Autodesk Inventor part; units mm, degrees
ref_plane "YZ Plane" through (0, 0, 0) normal (1, 0, 0) x (0, 1, 0)
ref_plane "XZ Plane" through (0, 0, 0) normal (0, 1, 0) x (-1, 0, 0)
ref_plane "XY Plane" through (0, 0, 0) normal (0, 0, 1) x (1, 0, 0)
sketch "Sketch1" plane through (0, 0, 0) normal (0, 0, 1) x (1, 0, 0)
  line L0 (-25, 0) -> (25, 0)
  line L1 (25, 0) -> (25, 394)
  line L2 (25, 394) -> (-25, 394)
  line L3 (-25, 394) -> (-25, 0)
  point P0 (0, 0)
  point P1 (0, 0)
  dimension "d0" = 394
  dimension "d1" = 50
extrude "Extrusion1" add sketch "Sketch1" along normal blind 3
sketch "Sketch2" plane through (0, 0, 0) normal (0, 0, -1) x (-1, 0, 0)
  line L0 (-22, 334) -> (-25, 334)
  line L1 (-22, 374) -> (-25, 374)
  line L2 (-22, 374) -> (-22, 354)
  line L3 (-25, 334) -> (-25, 354)
  line L4 (-25, 0) -> (-25, 394)
  line L5 (-22, 354) -> (-25, 354)
  line L6 (-25, 0) -> (-25, 394)
  line L7 (-25, 394) -> (25, 394)
  line L8 (-25, 354) -> (-25, 374)
  line L9 (-22, 354) -> (-22, 334)
  line L10 (-22, 374) -> (-25, 374)
  line L11 (-25, 374) -> (-25, 394)
  line L12 (-25, 394) -> (-22, 394)
  line L13 (-22, 394) -> (-22, 374)
  point P0 (0, 0)
  dimension "d4" = 20
  dimension "d10" = 20
  dimension "d55" = 60
  dimension "d56" = 20
extrude "Extrusion2" cut sketch "Sketch2" against normal blind 3 contours L5 L4 L1 L2 | L1 L4 L7 L13
sketch "Sketch3" plane through (0, 0, 0) normal (0, 0, -1) x (-1, 0, 0)
  line L0 (-25, 0) -> (-25, 354)
  line L1 (-25, 354) -> (-31, 354)
  line L2 (-31, 354) -> (-31, 336)
  line L3 (-29, 334) -> (-25, 334)
  line L4 (-25, 334) -> (-25, 354)
  line L5 (-31, 354) -> (-25, 354)
  line L6 (-25, 354) -> (-25, 374)
  line L7 (-25, 374) -> (-28, 374)
  line L8 (-31, 364) -> (-31, 354)
  line L9 (-31, 364) -> (-28, 374)
  line L10 (-28, 374) -> (-31, 374) construction
  arc A0 (-31, 336) -> (-29, 334) centre (-29, 336) ccw
  point P0 (0, 0)
  point P1 (-31, 334)
  dimension "d11" = 20
  dimension "d12" = 20
  dimension "d13" = 6
  dimension "d16" = 2
extrude "Extrusion3" add sketch "Sketch3" against normal blind 3
pattern_linear "Rectangular Pattern1" count 3 spacing 120 along (0, -1, 0) of "Extrusion2", "Extrusion3"
mirror "Mirror1" about plane through (0, 0, 0) normal (1, 0, 0) of "Extrusion2", "Rectangular Pattern1", "Extrusion3"
sketch "Sketch4" plane through (0, 0, 0) normal (0, 0, -1) x (-1, 0, 0)
  line L0 (-22, 384) -> (18.49, 384) construction
  line L1 (-22, 394) -> (22, 394)
  line L2 (-22, 394) -> (-22, 354)
  point P0 (0, 0)
  point P1 (-8, 384)
  point P2 (8, 384)
  dimension "d17" = 16
  dimension "d52" = 10
  dimension "d53" = 14
hole "Hole1" at (8, 384, 0) at (-8, 384, 0) direction (0, 0, 1) diameter 3.2 end through all
sketch "Sketch5" plane through (0, 0, 0) normal (0, 0, -1) x (-1, 0, 0)
  line L0 (-10, 0) -> (10, 0)
  line L1 (-10, 0) -> (-10, -6)
  line L2 (10, -6) -> (-10, -6)
  line L3 (10, 0) -> (10, -6)
  line L4 (25, 94) -> (25, 0)
  point P0 (0, 0)
  dimension "d48" = 6
  dimension "d50" = 20
  dimension "d51" = 15
extrude "Extrusion4" add sketch "Sketch5" against normal blind 3
sketch "Sketch6" plane through (0, 0, 0) normal (0, 0, -1) x (-1, 0, 0)
  line L0 (0, 36.6667) -> (0, 53.3333) construction
  line L1 (-10, 36.6667) -> (-10, 53.3333)
  line L2 (10, 53.3333) -> (10, 36.6667)
  arc A0 (-10, 36.6667) -> (10, 36.6667) centre (0, 36.6667) ccw
  arc A1 (10, 53.3333) -> (-10, 53.3333) centre (0, 53.3333) ccw
  line L3 (0, 343.6331) -> (0, 309.773) construction
  line L4 (-5.8349, 343.6331) -> (-5.8349, 309.773)
  line L5 (5.8349, 309.773) -> (5.8349, 343.6331)
  arc A2 (5.8349, 343.6331) -> (-5.8349, 343.6331) centre (0, 343.6331) ccw
  arc A3 (-5.8349, 309.773) -> (5.8349, 309.773) centre (0, 309.773) ccw
  line L6 (0, 243.6331) -> (0, 209.773) construction
  line L7 (-5.8349, 243.6331) -> (-5.8349, 209.773)
  line L8 (5.8349, 209.773) -> (5.8349, 243.6331)
  arc A4 (5.8349, 243.6331) -> (-5.8349, 243.6331) centre (0, 243.6331) ccw
  arc A5 (-5.8349, 209.773) -> (5.8349, 209.773) centre (0, 209.773) ccw
  line L9 (0, 143.6331) -> (0, 109.773) construction
  line L10 (-5.8349, 143.6331) -> (-5.8349, 109.773)
  line L11 (5.8349, 109.773) -> (5.8349, 143.6331)
  arc A6 (5.8349, 143.6331) -> (-5.8349, 143.6331) centre (0, 143.6331) ccw
  arc A7 (-5.8349, 109.773) -> (5.8349, 109.773) centre (0, 109.773) ccw
  point P0 (0, 0)
  point P1 (0, 45)
  point P2 (0, 326.7031)
  point P3 (0, 226.7031)
  point P4 (0, 126.7031)
  dimension "d28" = 10
  dimension "d29" = 45
  dimension "d43" = 100
extrude "Extrusion5" cut sketch "Sketch6" against normal blind 3
sketch "Sketch7" plane through (0, 0, 0) normal (0, 0, -1) x (-1, 0, 0)
  line L0 (-22, 10) -> (26.4852, 10) construction
  line L1 (-25, 0) -> (-25, 94)
  line L2 (-10, 0) -> (-25, 0)
  point P0 (0, 0)
  point P1 (-8, 10)
  point P2 (8, 10)
  dimension "d32" = 16
  dimension "d33" = 17
  dimension "d54" = 10
hole "Hole2" at (8, 10, 0) at (-8, 10, 0) direction (0, 0, 1) diameter 3.2 end through all
properties part number "Camera mounting back"
Geometry: final body of the model. Coordinates: model frame, mm. A direction names the side the tool comes from. Give positions to 0.01 mm unless a question says otherwise; leave off trailing zeros. Order: outer loops, then holes, each group sorted by start corner. A loop starts at its lowest first (then second) coordinate and runs counter-clockwise, first axis right, second up. Notation, with made-up numbers: (80.25, -4) -> (85.25, -4) arc R16 ccw to (85.25, 3) -> close; hole circle Ø1 at (85, -17). An arc over 180 degrees is marked (long way). Write each question's results on one line, items separated by ' | '. Start each with the question number.
1) First-contact query: pin 1 (1.5 mm diameter, centred on x = 24, z = 1.5, fed in from +Y); pin 2 (0.9 mm diameter, centred on x = 26, z = 1.5, fed in from +Y); pin 3 (2.5 mm diameter, centred on x = -8, y = 384, fed in from +Z). Flat tips, straight axial feed; report the tip coordinate or a pass-through.
2) Section C-C (y = 369.5). Return loops of the section in (x, z).
3) Section B-B (y = 327). Return loops of the section in (x, z).
4) Set-up query: faces 3 (the cylindrical face through (0.22, 26.67, 1.48)), 4 (the flat face through (0, 197, 3)). Return all of +Z, -Z, +X, -X, +Y, -Y with unobstructed straight access to the full face (end or side cutting, diameter ignored); none if empty.
5) Line query: line 1 (Y direction, x = 24, z = 2); line 2 (X direction, y = 10, z = 1.6); line 3 (X direction, y = 384, z = 1.7). Output: solid intervals per line, ascending. Write a range as from..to.
6) Section D-D (z = 1.2). Count the separate pieces of the cut face and the enclosed holes in it, then the cut area to 3 significant figures.
7) Section A-A (x = 0). Return loops of the section in (y, z).
8) Draft query along Y for faces 1 (the flat face through (0, 197, 0)), 2 (the cylindrical face through (-0.22, 63.33, 1.48)). Return one class per face: pulls with the +Y half, pulls with the -Y half, needs draft (parallel to the pull), parting line crosses it, or undercut.
Calculated:
1) pin 1: y = 354 | pin 2: y = 374 | pin 3: through
2) outline: (-29.35, 0) -> (-25, 0) -> (-25, 3) -> (-29.35, 3) -> close; (-22, 0) -> (22, 0) -> (22, 3) -> (-22, 3) -> close; (25, 0) -> (29.35, 0) -> (29.35, 3) -> (25, 3) -> close
3) outline: (-25, 0) -> (-5.83, 0) -> (-5.83, 3) -> (-25, 3) -> close; (5.83, 0) -> (25, 0) -> (25, 3) -> (5.83, 3) -> close
4) face 3: +Z, -Z | face 4: +Z, +X, -X, +Y, -Y
5) line 1: 0..114, 154..234, 274..354 | line 2: -25..-9.6, -6.4..6.4, 9.6..25 | line 3: -22..-9.6, -6.4..6.4, 9.6..22
6) separate pieces: 1 | enclosed holes: 8 | area: 18,300 mm2
7) outline: (-6, 0) -> (26.67, 0) -> (26.67, 3) -> (-6, 3) -> close; (63.33, 0) -> (103.94, 0) -> (103.94, 3) -> (63.33, 3) -> close; (149.47, 0) -> (203.94, 0) -> (203.94, 3) -> (149.47, 3) -> close; (249.47, 0) -> (303.94, 0) -> (303.94, 3) -> (249.47, 3) -> close; (349.47, 0) -> (394, 0) -> (394, 3) -> (349.47, 3) -> close
8) face 1: needs draft | face 2: undercut
